```python
from build123d import *

# Parameters (mm, degrees)
F0_W          = 244.475
F0_H          = 422.275
F1_DEPTH      = 6.35
F0_W_2        = 269.875
F0_H_2        = 447.675
F2_DEPTH      = 127
F2_DEPTH_BACK = 25.4
F3_W          = 76.2
F3_H          = 422.275
F4_DEPTH      = 19.05
F6_DEPTH      = 25.4


with BuildPart() as f1:
    # F0 (on Top) → F1 (new body)
    with BuildSketch(Plane.XY):
        with Locations((-122.2375, -211.1375)):
            Rectangle(F0_W, F0_H)
    extrude(amount=-F1_DEPTH)

    # F0 (on Top) → F2 (join, two sides)
    with BuildSketch(Plane.XY) as f2_sk:
        with Locations((-122.2375, -211.1375)):
            Rectangle(F0_W_2, F0_H_2)
        with Locations((-122.2375, -211.1375)):
            Rectangle(F0_W, F0_H, mode=Mode.SUBTRACT)
    extrude(amount=F2_DEPTH)
    extrude(f2_sk.sketch, amount=-F2_DEPTH_BACK)

    # F3 (on face) → F4 (join, through all)
    with BuildSketch(Plane(origin=(0, 0, -6.35), x_dir=(1, 0, 0), z_dir=(0, 0, -1))):
        with Locations((-130.175, 211.1375)):
            Rectangle(F3_W, F3_H)
    extrude(amount=F4_DEPTH)

    # F5 (on face) → F6 (cut)
    with BuildSketch(Plane.XZ.offset(434.975)):
        with BuildLine():
            Line((-38.1, 158.75), (-206.375, 158.75))
            ThreePointArc((-206.375, 158.75), (-200.788921, 142.139157), (-191.961107, 127))
            Line((-191.961107, 127), (-52.513893, 127))
            ThreePointArc((-52.513893, 127), (-43.686079, 142.139157), (-38.1, 158.75))
        make_face()
        with BuildLine():
            Line((-52.513893, 127), (-191.961107, 127))
            ThreePointArc((-191.961107, 127), (-122.2375, 91.532849), (-52.513893, 127))
        make_face()
    extrude(amount=-F6_DEPTH, mode=Mode.SUBTRACT)


solid = f1.part
```
Can you work these out from the model? Positions are in its coordinate system, mm. A direction names the side the tool comes from. Round coordinates to 2 decimals unless told otherwise and drop trailing zeros. Loops run counter-clockwise (first coordinate to the right, second up) from the corner with the lowest first, then second, coordinate; pieces in that order, holes last.
Item 1: Suppose I cut it at A-A, the plane z = 75.5. Write out the boundary of the cut face in (x, y) (3 decimals), then the cut area to 3 significant figures.
Item 2: If we mould it in two halves opening along X, with no side actions, what happens to faces 1 (the flat face through (-124, 12.7, 52)), 2 (the flat face through (-257.175, -214, 52)), 3 (the flat face through (-124, 0, 63)), 4 (the flat face through (12.7, -214, 52))? For each: +X half, -X half, draft (parallel to the pull), parting line (faces both ways), or undercut.
Item 3: Will these pins go through, and if not, where does the flat tip stop? pin 1 Ø1.5 at (x, z) = (-147, 106.5) entering from -Y; pin 2 Ø3 at (x, y) = (-30, -209) entering from +Z.
Item 4: Which directions (+Z, -Z, +X, -X, +Y, -Y) give clear straight access to the entire face, cutting with the end or side of a thin tool? Please do faces 5 (the cylindrical face through (-123.37, -428.71, 91.54)), 6 (the flat face through (-124, -434.975, 52)), 7 (the flat face through (-207, -422.275, -16)), 8 (the flat face through (-253, -177, 127)), 9 (the flat face through (0, -214, 63)).
Item 5: Suppose I cut it at B-B, the plane y = -51.5. Write out the boundary of the cut face in (x, z) (3 decimals).
Item 6: Please list where these lines run through material, in increasing order: L1, parallel to X at y = -113, z = 119 (3 decimals); L2, parallel to Y at x = -33.5, z = 85.5 (3 decimals); L3, parallel to X at y = -298, z = -8 (3 decimals).
Item 7: Suppose I cut it at D-D, the plane z = 96. Write out the boundary of the cut face in (x, y) (3 decimals).
Item 8: Suppose I cut it at C-C, the plane x = -23.5. Write out the boundary of the cut face in (y, z) (3 decimals).
Reported:
1. outline: (-257.175, -434.975) - (12.7, -434.975) - (12.7, 12.7) - (-257.175, 12.7) - close; hole (-244.475, -422.275) - (0, -422.275) - (0, 0) - (-244.475, 0) - close
1. area: 17,600 mm2
2. face 1: draft
2. face 2: -X half
2. face 3: undercut
2. face 4: +X half
3. pin 1: stops at y = 0
3. pin 2: stops at z = 0
4. face 5: +Z, -Y
4. face 6: +Z, -Z, +X, -X, -Y
4. face 7: -Z
4. face 8: +Z, +X, -X, +Y, -Y
4. face 9: +Z
5. outline: (-257.175, -25.4) - (-244.475, -25.4) - (-244.475, -6.35) - (-168.275, -6.35) - (-168.275, -25.4) - (-92.075, -25.4) - (-92.075, -6.35) - (0, -6.35) - (0, -25.4) - (12.7, -25.4) - (12.7, 127) - (0, 127) - (0, 0) - (-244.475, 0) - (-244.475, 127) - (-257.175, 127) - close
6. L1: x = -257.175 to -244.475, 0 to 12.7
6. L2: y = -434.975 to -422.275, 0 to 12.7
6. L3: x = -257.175 to -244.475, -168.275 to -92.075, 0 to 12.7
7. outline: (-257.175, -434.975) - (-149.638, -434.975) - (-149.638, -422.275) - (-244.475, -422.275) - (-244.475, 0) - (0, 0) - (0, -422.275) - (-94.837, -422.275) - (-94.837, -434.975) - (12.7, -434.975) - (12.7, 12.7) - (-257.175, 12.7) - close
8. outline: (-434.975, -25.4) - (-422.275, -25.4) - (-422.275, -6.35) - (0, -6.35) - (0, -25.4) - (12.7, -25.4) - (12.7, 127) - (0, 127) - (0, 0) - (-422.275, 0) - (-422.275, 127) - (-434.975, 127) - close
